Design review of the part shown in the three views and the two pictorial views. Dimensions are in mm from the part's minimum x, y and z. A direction names the side the tool comes from. Give positions to 0.01 mm unless a question says otherwise; leave off trailing zeros. Order: outer loops, then holes, each group sorted by start corner. A loop starts at its lowest first (then second) coordinate and runs counter-clockwise, first axis right, second up. Notation, with made-up numbers: M 28,75 L 72,75 A18 ccw 72,106 Z; hole C 88.5,17.5 d11. An arc over 180 degrees is marked long. Answer as a JSON object with one key per item and string values.
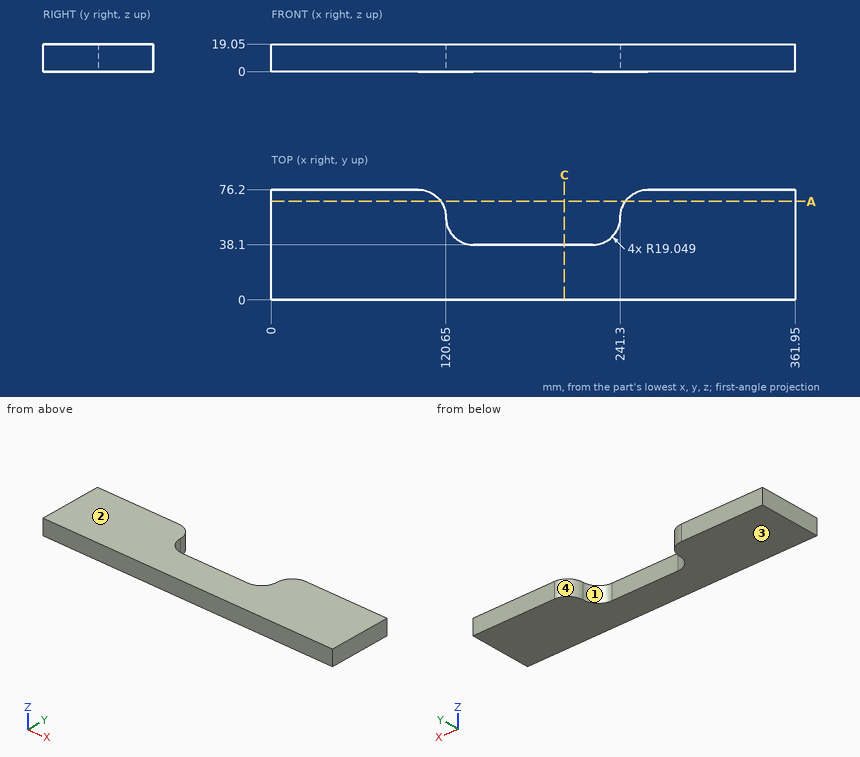
(1) We need section A-A (y = 68). Write out the cut boundary in (x, z), plus the area to 3 significant figures.
Checked values:
{"outline": "M 0,0 L 117.26,0 L 117.26,19.05 L 0,19.05 Z; M 244.69,0 L 361.95,0 L 361.95,19.05 L 244.69,19.05 Z", "area": "4,470 mm^2"}
(2) Draft analysis for pull direction X (two halves, no side actions). For the marked faces 1 and 2, state which applies: +X half, -X half, draft (parallel to the pull), parting line (faces both ways), or undercut.
Checked values:
{"face 1": "undercut", "face 2": "draft"}
(3) To check wall thickness, follow L1, parallel to X at y = 57.5, z = 5.5; L2, parallel to Y at x = 182.5, z = 13.5; L3, parallel to X at y = 65, z = 17.5. State the ranges of each line that lie inside material, in increasing order. Write a range as from..to.
Checked values:
{"L1": "x = 0..120.65, 241.3..361.95", "L2": "y = 0..38.1", "L3": "x = 0..118.96, 242.99..361.95"}
(4) Tool access review of the marked faces 3 and 4: name each direction out of +Z, -Z, +X, -X, +Y, -Y from which nothing blocks a thin tool from reaching the whole face with its end or side.
Checked values:
{"face 3": "-Z, +X, -X, +Y, -Y", "face 4": "+Z, -Z, +Y"}
(5) Insertion check: pin 1 (3 mm diameter, centred on x = 260.5, z = 3, fed in from -Y). The pin has a flat end and moves straight along its axis. Give the tip position at first contact, or say it passes through.
Checked values:
{"pin 1": "stops at y = 0"}
(6) We need section C-C (x = 202.5). Write out the cut boundary in (y, z).
Checked values:
{"outline": "M 0,0 L 38.1,0 L 38.1,19.05 L 0,19.05 Z"}
